```python
from build123d import *

# Parameters (mm, degrees)
F1_DEPTH = 50
F2_R     = 5.08
F4_D     = 5


with BuildPart() as f1:
    # F0 (on Right) → F1 (new body)
    with BuildSketch(Plane.YZ):
        Polygon((1.439528, 14.019234), (1.439528, 11.019234), (-7.985472, 11.019234), (-7.985472, 6.019234), (17.014528, 6.019234), (17.014528, 11.019234), (7.589528, 11.019234), (7.589528, 14.019234), align=None)
    extrude(amount=F1_DEPTH)

    # F2
    f2_edges = [f1.edges().sort_by_distance(p)[0] for p in [
        (50, 17.014528, 8.519234),
        (50, -7.985472, 8.519234),
        (0, 17.014528, 8.519234),
        (0, -7.985472, 8.519234),
    ]]
    fillet(f2_edges, radius=F2_R)

    # F4 (through all)
    with Locations(Plane.XY.offset(14.019234)):
        with Locations((16.666667, 4.514528), (33.333333, 4.514528)):
            Hole(F4_D / 2)


solid = f1.part
```
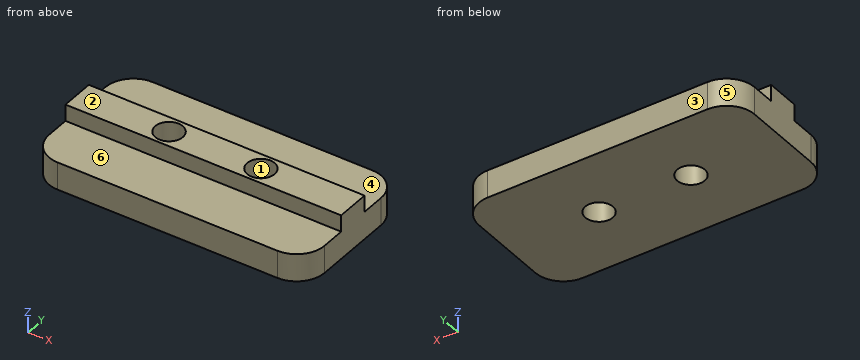
Can you work these out from the model? Positions are in its coordinate system, mm. Face numbers are marked on the shaded views. A direction names the side the tool comes from. Give positions to 0.01 mm unless a question says otherwise; leave off trailing zeros. Loops run counter-clockwise (first coordinate to the right, second up) from the corner with the lowest first, then second, coordinate; pieces in that order, holes last. Notation, with made-up numbers: M -32,69.5 L 15,69.5 A28 cw 15,96.5 Z; hole C 12.25,82.25 d5. An arc over 180 degrees is marked long. Answer in a Markdown table with one row per item.
1. Which directions (+Z, -Z, +X, -X, +Y, -Y) give clear straight access to the entire face, cutting with the end or side of a thin tool? Please do the marked faces 4, 5 and 6.
Taken from the geometry:
| item | result |
|---|---|
| face 4 | +Z, +X, -X, +Y |
| face 5 | +Z, -Z, -X, +Y |
| face 6 | +Z, +X, -X, -Y |
2. Suppose I cut it at D-D on x = 32.5. Write out the boundary of the cut face in (y, z), plus the area to 3 significant figures.
Taken from the geometry:
| item | result |
|---|---|
| outline | M -7.99,6.02 L 2.16,6.02 L 2.16,14.02 L 1.44,14.02 L 1.44,11.02 L -7.99,11.02 Z; M 6.87,6.02 L 17.01,6.02 L 17.01,11.02 L 7.59,11.02 L 7.59,14.02 L 6.87,14.02 Z |
| area | 106 mm² |
3. Suppose I cut it at A-A on y = 3.75. Write out the boundary of the cut face in (x, z).
Taken from the geometry:
| item | result |
|---|---|
| outline | M 0,6.02 L 14.29,6.02 L 14.29,14.02 L 0,14.02 Z; M 19.05,6.02 L 30.95,6.02 L 30.95,14.02 L 19.05,14.02 Z; M 35.71,6.02 L 50,6.02 L 50,14.02 L 35.71,14.02 Z |
4. If I drill on line 1 along X through (y, z) = (6.25, 7); line 2 along X through (y, z) = (3.5, 11.25); line 3 along Y through (x, z) = (11.5, 13.5), over which ranges is the centre line in solid material (lowest first)?
Taken from the geometry:
| item | result |
|---|---|
| line 1 | x = 0 to 14.87, 18.47 to 31.53, 35.13 to 50 |
| line 2 | x = 0 to 14.38, 18.95 to 31.05, 35.62 to 50 |
| line 3 | y = 1.44 to 7.59 |
5. For pin 1 Ø2.5 at (x, z) = (30.5, 13) entering from +Y; pin 2 Ø4.5 at (x, y) = (17, 10) entering from +Z; pin 3 Ø1.5 at (x, z) = (36, 13) entering from -Y, each with a flat end and sliding along its axis, tell me the tip position at first contact or that it passes through.
Taken from the geometry:
| item | result |
|---|---|
| pin 1 | stops at y = 7.59 |
| pin 2 | stops at z = 11.02 |
| pin 3 | stops at y = 1.44 |
6. Suppose I cut it at B-B on x = 10. Write out the boundary of the cut face in (y, z), plus the area to 3 significant figures.
Taken from the geometry:
| item | result |
|---|---|
| outline | M -7.99,6.02 L 17.01,6.02 L 17.01,11.02 L 7.59,11.02 L 7.59,14.02 L 1.44,14.02 L 1.44,11.02 L -7.99,11.02 Z |
| area | 143 mm² |
7. Thinking about a two-plate mould opening in Y: for the marked faces 1, 2 and 3, which applies, released by +Y, released by -Y, zero draft, split by the parting line, or undercut?
Taken from the geometry:
| item | result |
|---|---|
| face 1 | undercut |
| face 2 | zero draft |
| face 3 | released by +Y |
8. Suppose I cut it at C-C on z = 11.5. Write out the boundary of the cut face in (x, y).
Taken from the geometry:
| item | result |
|---|---|
| outline | M 0,1.44 L 50,1.44 L 50,7.59 L 0,7.59 Z; hole C 16.67,4.51 d5; hole C 33.33,4.51 d5 |
